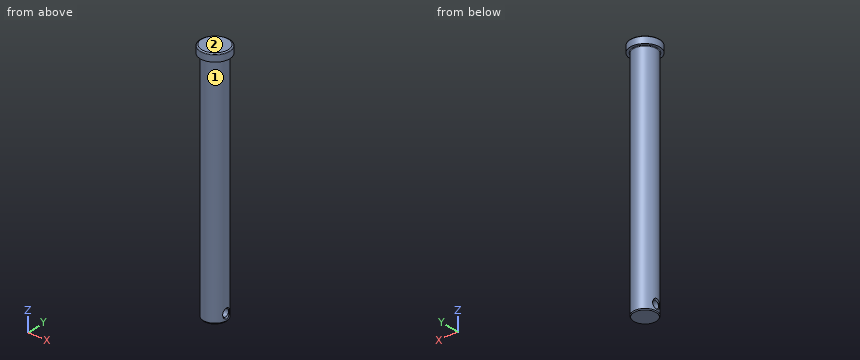
```python
from build123d import *

# Parameters (mm, degrees)
CUT_EXTRUDE1_DEPTH      = 69.504934844
CUT_EXTRUDE1_DEPTH_BACK = 69.504934844
SKETCH3_R               = 1.9812
FILLET1_R               = 0.3175


with BuildPart() as part:
    # Sketch2 → Revolve1 (revolve)
    with BuildSketch(Plane(origin=(0, 0, 0), x_dir=(0, 0, -1), z_dir=(1, 0, 0)), mode=Mode.PRIVATE) as revolve1_sk:
        Polygon((63.5, 6.0325), (63.5, 0), (-67.564, 0), (-67.564, 7.1882), (-67.094729701, 8.001), (-63.5, 8.001), (-63.5, 6.35), (62.950073869, 6.35), align=None)
    revolve(revolve1_sk.sketch.rotate(Axis((0, 0, 63.5), (0, 0, -1)), 90), axis=Axis((0, 0, 63.5), (0, 0, -1)))

    # Sketch3 → Cut-Extrude1 (cut, two sides: drawn at the far end of the back side and taken through both)
    with BuildSketch(Plane(origin=(0, 0, 0), x_dir=(0, 0, -1), z_dir=(1, 0, 0)).offset(-CUT_EXTRUDE1_DEPTH_BACK)):
        with Locations((59.5122, 0)):
            Circle(SKETCH3_R)
    extrude(amount=CUT_EXTRUDE1_DEPTH + CUT_EXTRUDE1_DEPTH_BACK, mode=Mode.SUBTRACT)

    # Fillet1
    fillet1_edges = [part.edges().sort_by_distance(p)[0] for p in [
        (-8.001, 0, 67.094729701),
        (-6.35, 0, 63.5),
    ]]
    fillet(fillet1_edges, radius=FILLET1_R)

    # Sketch4 → Cut-Revolve1 (revolve, cut)
    with BuildSketch(Plane(origin=(0, 0, 0), x_dir=(1, 0, 0), z_dir=(0, 1, 0)), mode=Mode.PRIVATE) as cut_revolve1_sk:
        Polygon((6.35, 59.5122), (6.35, 56.8706), (3.7084, 59.5122), align=None)
        Polygon((-6.35, 56.8706), (-3.7084, 59.5122), (-6.35, 59.5122), align=None)
    revolve(cut_revolve1_sk.sketch.rotate(Axis((6.35, 0, -59.5122), (-1, 0, 0)), 180), axis=Axis((6.35, 0, -59.5122), (-1, 0, 0)), mode=Mode.SUBTRACT)


solid = part.part
```
Verification items for the finished model (mm, model axes). Face numbers are marked on the shaded views. A direction names the side the tool comes from. Coordinates: 2 decimals unless noted, no trailing zeros. Write each loop counter-clockwise with the first axis right and the second up, starting at its lowest first coordinate (ties: lowest second). Pieces come first, ordered by that corner, then holes. Notation, with made-up numbers: (67.5, 10) - (112.5, 10) arc R12 cw to (112.5, 17) - close; hole circle Ø8 at (-17, 38.25). An arc over 180 degrees is marked (long way). Write item = value, one per line.
Q1. Access from +Z, -Z, +X, -X, +Y, -Y to the whole of each face (thin tool, end or side, straight path). Record for the marked faces 1 and 2.
Answer:
face_1 = -Z
face_2 = +Z, +X, -X, +Y, -Y
Q2. Material ranges on L1, parallel to Z at x = -2.75, y = -0.25; L2, parallel to Z at x = 2.5, y = -6.75; L3, parallel to Y at x = 2, z = -55, recorded low to high. Write a range as from..to.
Answer:
L1 = -63.5..-61.48, -57.55..67.56
L2 = 63.5..67.56
L3 = -6.03..6.03
Q3. Cross-section at A-A (z = -48.5). Enter the section's corners in (x, y), plus the area to 3 significant figures.
Answer:
outline = circle Ø12.7 at (0, 0)
area = 127 mm²
Q4. Go/stop test with flat-tipped pins: pin 1 Ø8 at (y, z) = (1.5, 44.5) entering from -X; pin 2 Ø8 at (y, z) = (1.5, -14.5) entering from +X; pin 3 Ø1.5 at (x, z) = (3.5, -40.5) entering from +Y. Record where each tip stops, or that it passes through.
Answer:
pin_1 = -6.35
pin_2 = 6.35
pin_3 = 5.72
